Here's how the part is built. I have some questions about the finished solid (model axes, mm). A direction names the side the tool comes from. Round coordinates to 2 decimals unless told otherwise and drop trailing zeros. Loops run counter-clockwise (first coordinate to the right, second up) from the corner with the lowest first, then second, coordinate; pieces in that order, holes last. Notation, with made-up numbers: M -18.75,4 L 7.25,4 A31 cw 7.25,34 Z; hole C -9.5,-1.5 d8. An arc over 180 degrees is marked long. Use a Markdown table: item, result.
```python
from build123d import *

# Parameters (mm, degrees)
SKETCH_1_W           = 40
SKETCH_1_H           = 40
EXTRUDE_1_DEPTH      = 9
SKETCH_2_W           = 8
SKETCH_2_H           = 40
CUT_EXTRUDE_1_DEPTH  = 3.5
SKETCH_3_R           = 1.15
CUT_EXTRUDE_2_DEPTH  = 58.280013966
SKETCH_4_R           = 2
CUT_EXTRUDE_3_DEPTH  = 2.4
SKETCH_5_R           = 1.2
CUT_EXTRUDE_4_DEPTH  = 58.280013966
SKETCH_6_R           = 2
CUT_EXTRUDE_5_DEPTH  = 5.7
SKETCH_7_W           = 13.47912662
SKETCH_7_H           = 15
CUT_EXTRUDE_6_DEPTH  = 3.5
SKETCH_12_W          = 4
SKETCH_12_H          = 40
SKETCH_12_W_2        = 21.6
SKETCH_12_H_2        = 12
SKETCH_12_H_3        = 14
CUT_EXTRUDE_11_DEPTH = 4
FILLET_3_R           = 2
SKETCH_15_R          = 3.6
CUT_EXTRUDE_13_DEPTH = 4
SKETCH_16_W          = 5
SKETCH_16_H          = 7
CUT_EXTRUDE_14_DEPTH = 3.5
SKETCH_17_R          = 1.5
CUT_EXTRUDE_15_DEPTH = 3.5
FILLET_5_R           = 2
SKETCH_18_W          = 10
SKETCH_18_H          = 40
CUT_EXTRUDE_16_DEPTH = 3.5


with BuildPart() as part:
    # 草图1 → 凸台-拉伸1 (new body)
    with BuildSketch(Plane(origin=(0, 0, 0), x_dir=(1, 0, 0), z_dir=(0, 1, 0))):
        with Locations((20, -20)):
            Rectangle(SKETCH_1_W, SKETCH_1_H)
    extrude(amount=EXTRUDE_1_DEPTH)

    # 草图2 → 切除-拉伸1 (cut)
    with BuildSketch(Plane(origin=(0, 9, 0), x_dir=(1, 0, 0), z_dir=(0, 1, 0))):
        with Locations((20, -20)):
            Rectangle(SKETCH_2_W, SKETCH_2_H)
    extrude(amount=-CUT_EXTRUDE_1_DEPTH, mode=Mode.SUBTRACT)

    # 草图3 → 切除-拉伸2 (cut, through all)
    with BuildSketch(Plane(origin=(0, 0, 0), x_dir=(-1, 0, 0), z_dir=(0, -1, 0))):
        with Locations(Location((-20, -22.5, 0), (0, 0, 90))):
            Circle(SKETCH_3_R)
        with Locations(Location((-20, -17.5, 0), (0, 0, 90))):
            Circle(SKETCH_3_R)
    extrude(amount=-CUT_EXTRUDE_2_DEPTH, mode=Mode.SUBTRACT)

    # 草图4 → 切除-拉伸3 (cut)
    with BuildSketch(Plane(origin=(0, 0, 0), x_dir=(-1, 0, 0), z_dir=(0, -1, 0))):
        with Locations(Location((-20, -22.5, 0), (0, 0, 90))):
            Circle(SKETCH_4_R)
        with Locations(Location((-20, -17.5, 0), (0, 0, 90))):
            Circle(SKETCH_4_R)
    extrude(amount=-CUT_EXTRUDE_3_DEPTH, mode=Mode.SUBTRACT)

    # 草图5 → 切除-拉伸4 (cut, through all)
    with BuildSketch(Plane(origin=(0, 9, 0), x_dir=(1, 0, 0), z_dir=(0, 1, 0))):
        with Locations(Location((25.8, -20, 0), (0, 0, 270))):
            Circle(SKETCH_5_R)
        with Locations(Location((30.8, -20, 0), (0, 0, 270))):
            Circle(SKETCH_5_R)
    extrude(amount=-CUT_EXTRUDE_4_DEPTH, mode=Mode.SUBTRACT)

    # 草图6 → 切除-拉伸5 (cut)
    with BuildSketch(Plane(origin=(0, 9, 0), x_dir=(1, 0, 0), z_dir=(0, 1, 0))):
        with Locations(Location((30.8, -20, 0), (0, 0, 270))):
            Circle(SKETCH_6_R)
        with Locations(Location((25.8, -20, 0), (0, 0, 270))):
            Circle(SKETCH_6_R)
    extrude(amount=-CUT_EXTRUDE_5_DEPTH, mode=Mode.SUBTRACT)

    # 草图7 → 切除-拉伸6 (cut)
    with BuildSketch(Plane(origin=(0, 9, 0), x_dir=(1, 0, 0), z_dir=(0, 1, 0))):
        with Locations((9.26043669, -21.5)):
            Rectangle(SKETCH_7_W, SKETCH_7_H)
    extrude(amount=-CUT_EXTRUDE_6_DEPTH, mode=Mode.SUBTRACT)

    # 草图12 → 切除-拉伸11 (cut)
    with BuildSketch(Plane(origin=(0, 0, 0), x_dir=(-1, 0, 0), z_dir=(0, -1, 0))):
        with Locations((-4.2, -20)):
            Rectangle(SKETCH_12_W, SKETCH_12_H)
        with Locations((-35.8, -20)):
            Rectangle(SKETCH_12_W, SKETCH_12_H)
        with Locations((-20, -6)):
            Rectangle(SKETCH_12_W_2, SKETCH_12_H_2)
        with Locations((-20, -33)):
            Rectangle(SKETCH_12_W_2, SKETCH_12_H_3)
    extrude(amount=-CUT_EXTRUDE_11_DEPTH, mode=Mode.SUBTRACT)

    # 圆角3
    fillet_3_edges = [part.edges().sort_by_distance(p)[0] for p in [
        (30.8, 2, 12),
        (9.2, 2, 12),
        (9.2, 2, 26),
        (30.8, 2, 26),
    ]]
    fillet(fillet_3_edges, radius=FILLET_3_R)

    # 草图15 → 切除-拉伸13 (cut)
    with BuildSketch(Plane(origin=(0, 5.5, 0), x_dir=(1, 0, 0), z_dir=(0, 1, 0))):
        with Locations(Location((20, -8.5, 0), (0, 0, 270))):
            Circle(SKETCH_15_R)
    extrude(amount=-CUT_EXTRUDE_13_DEPTH, mode=Mode.SUBTRACT)

    # 草图16 → 切除-拉伸14 (cut)
    with BuildSketch(Plane(origin=(0, 9, 0), x_dir=(1, 0, 0), z_dir=(0, 1, 0))):
        with Locations((11.5, -32.5)):
            Rectangle(SKETCH_16_W, SKETCH_16_H)
    extrude(amount=-CUT_EXTRUDE_14_DEPTH, mode=Mode.SUBTRACT)

    # 草图17 → 切除-拉伸15 (cut)
    with BuildSketch(Plane(origin=(0, 5.5, 0), x_dir=(1, 0, 0), z_dir=(0, 1, 0))):
        with Locations(Location((11.5, -34, 0), (0, 0, 270))):
            Circle(SKETCH_17_R)
    extrude(amount=-CUT_EXTRUDE_15_DEPTH, mode=Mode.SUBTRACT)

    # 圆角5
    fillet_5_edges = [part.edges().sort_by_distance(p)[0] for p in [
        (9, 7.25, 36),
        (14, 7.25, 36),
        (2.52087338, 7.25, 29),
        (2.52087338, 7.25, 14),
    ]]
    fillet(fillet_5_edges, radius=FILLET_5_R)

    # 草图18 → 切除-拉伸16 (cut)
    with BuildSketch(Plane(origin=(0, 9, 0), x_dir=(1, 0, 0), z_dir=(0, 1, 0))):
        with Locations((32, -20)):
            Rectangle(SKETCH_18_W, SKETCH_18_H)
    extrude(amount=-CUT_EXTRUDE_16_DEPTH, mode=Mode.SUBTRACT)


solid = part.part
```
Q1. Will these pins go through, and if not, where does the flat tip stop? P1, Ø1.2, axis at x = 18.5, y = 1.5, coming from the -Z side; P2, Ø2.5, axis at x = 20, z = 22.5, coming from the -Y side; P3, Ø3, axis at x = 11.5, z = 30.5, coming from the -Y side.
Return value:
| item | result |
|---|---|
| P1 | stops at z = 12 |
| P2 | stops at y = 2.4 |
| P3 | stops at y = 4 |
Q2. For faces 5 (the flat face through (24, 3.3, 20)), 6 (the flat face through (20, 4, 33)), 7 (the flat face through (33.8, 2, 20)), 8 (the flat face through (27, 7, 31)), which set-ups out of +Z, -Z, +X, -X, +Y, -Y let a thin tool reach every point of the face, with its end or its side?
Return value:
| item | result |
|---|---|
| face 5 | +Y |
| face 6 | +Z, -Y |
| face 7 | +Z, -Z, -Y |
| face 8 | +Z, -Z, +Y |
Q3. We'd pull the mould along Z, two halves only. Please class faces 1 (the cylindrical face through (9.77, 2.03, 11.4)), 2 (the cylindrical face through (30.23, 2.03, 26.6)), 3 (the flat face through (11.5, 7.3, 36)), 4 (the flat face through (20, 0, 20)): pulls with the +Z half, pulls with the -Z half, needs draft (parallel to the pull), parting line crosses it, or undercut.
Return value:
| item | result |
|---|---|
| face 1 | pulls with the -Z half |
| face 2 | pulls with the +Z half |
| face 3 | undercut |
| face 4 | needs draft |
Q4. Imagine slicing it at A-A, the plane y = 1. Please give me the cut outline in (x, z), then the cut area to 3 significant figures.
Return value:
| item | result |
|---|---|
| outline | M 0,0 L 2.2,0 L 2.2,40 L 0,40 Z; M 6.2,0 L 9.2,0 L 9.2,10 A2 cw 11.2,12 L 28.8,12 A2 cw 30.8,10 L 30.8,0 L 33.8,0 L 33.8,40 L 30.8,40 L 30.8,28 A2 cw 28.8,26 L 11.2,26 A2 cw 9.2,28 L 9.2,40 L 6.2,40 Z; M 37.8,0 L 40,0 L 40,40 L 37.8,40 Z; hole C 20,17.5 d4; hole C 20,22.5 d4; hole C 25.8,20 d2.4; hole C 30.8,20 d2.4 |
| area | 688 mm^2 |
Q5. Imagine slicing it at C-C, the plane z = 8.5. Please give me the cut outline in (x, y), then the cut area to 3 significant figures.
Return value:
| item | result |
|---|---|
| outline | M 0,0 L 2.2,0 L 2.2,4 L 6.2,4 L 6.2,0 L 9.2,0 L 9.2,4 L 16.4,4 L 16.4,5.5 L 16,5.5 L 16,9 L 0,9 Z; M 23.6,4 L 30.8,4 L 30.8,0 L 33.8,0 L 33.8,4 L 37.8,4 L 37.8,0 L 40,0 L 40,9 L 37,9 L 37,5.5 L 27,5.5 L 27,9 L 24,9 L 24,5.5 L 23.6,5.5 Z |
| area | 168 mm^2 |
Q6. Imagine slicing it at B-B, the plane x = 20. Please give me the cut outline in (y, z), then the cut area to 3 significant figures.
Return value:
| item | result |
|---|---|
| outline | M 0,12 L 1.5,12 L 1.5,12.1 L 5.5,12.1 L 5.5,16.35 L 2.4,16.35 L 2.4,15.5 L 0,15.5 Z; M 0,19.5 L 2.4,19.5 L 2.4,18.65 L 5.5,18.65 L 5.5,21.35 L 2.4,21.35 L 2.4,20.5 L 0,20.5 Z; M 0,24.5 L 2.4,24.5 L 2.4,23.65 L 5.5,23.65 L 5.5,40 L 4,40 L 4,26 L 0,26 Z; M 4,0 L 5.5,0 L 5.5,4.9 L 4,4.9 Z |
| area | 71.5 mm^2 |
Q7. I need wall thicknesses on line 1 (X direction, y = 2.5, z = 20); line 2 (X direction, y = 6, z = 4); line 3 (X direction, y = 6.25, z = 33.5). Which ranges of each line are inside material? Lowest first, please. Write a range as from..to.
Return value:
| item | result |
|---|---|
| line 1 | x = 0..2.2, 6.2..24.6, 27..29.6, 32..33.8, 37.8..40 |
| line 2 | x = 0..16, 24..27, 37..40 |
| line 3 | x = 0..9, 14..16, 24..27, 37..40 |
Q8. Imagine slicing it at D-D, the plane x = 25.8. Please give me the cut outline in (y, z).
Return value:
| item | result |
|---|---|
| outline | M 0,12 L 4,12 L 4,0 L 9,0 L 9,18 L 3.3,18 L 3.3,18.8 L 0,18.8 Z; M 0,21.2 L 3.3,21.2 L 3.3,22 L 9,22 L 9,40 L 4,40 L 4,26 L 0,26 Z |
